```python
from build123d import *

# Parameters (mm, degrees)
BOSS_EXTRUDE1_DEPTH = 24
SKETCH2_R           = 5
BOSS_EXTRUDE2_DEPTH = 16
FILLET1_R           = 2
SKETCH4_W           = 5.41
SKETCH4_H           = 3.8
CUT_EXTRUDE1_DEPTH  = 20


with BuildPart() as part:
    # Sketch1 → Boss-Extrude1 (new body)
    with BuildSketch(Plane(origin=(0, 0, 0), x_dir=(0, 0, -1), z_dir=(1, 0, 0))):
        with BuildLine():
            Line((1.8, 31.882308546), (9.77686398, 36.487753113))
            Line((9.77686398, 36.487753113), (14.382308546, 28.510889132))
            ThreePointArc((14.382308546, 28.510889132), (15.7, 27.193197679), (17.5, 26.710889132))
            Line((17.5, 26.710889132), (26.710889132, 26.710889132))
            Line((26.710889132, 26.710889132), (26.710889132, 17.5))
            ThreePointArc((26.710889132, 17.5), (27.193197679, 15.7), (28.510889132, 14.382308546))
            Line((28.510889132, 14.382308546), (36.487753113, 9.77686398))
            Line((36.487753113, 9.77686398), (31.882308546, 1.8))
            ThreePointArc((31.882308546, 1.8), (31.4, 0), (31.882308546, -1.8))
            Line((31.882308546, -1.8), (36.487753113, -9.77686398))
            Line((36.487753113, -9.77686398), (28.510889132, -14.382308546))
            ThreePointArc((28.510889132, -14.382308546), (27.193197679, -15.7), (26.710889132, -17.5))
            Line((26.710889132, -17.5), (26.710889132, -26.710889132))
            Line((26.710889132, -26.710889132), (17.5, -26.710889132))
            ThreePointArc((17.5, -26.710889132), (15.7, -27.193197679), (14.382308546, -28.510889132))
            Line((14.382308546, -28.510889132), (9.77686398, -36.487753113))
            Line((9.77686398, -36.487753113), (1.8, -31.882308546))
            ThreePointArc((1.8, -31.882308546), (0, -31.4), (-1.8, -31.882308546))
            Line((-1.8, -31.882308546), (-9.77686398, -36.487753113))
            Line((-9.77686398, -36.487753113), (-14.382308546, -28.510889132))
            ThreePointArc((-14.382308546, -28.510889132), (-15.7, -27.193197679), (-17.5, -26.710889132))
            Line((-17.5, -26.710889132), (-26.710889132, -26.710889132))
            Line((-26.710889132, -26.710889132), (-26.710889132, -17.5))
            ThreePointArc((-26.710889132, -17.5), (-27.193197679, -15.7), (-28.510889132, -14.382308546))
            Line((-28.510889132, -14.382308546), (-36.487753113, -9.77686398))
            Line((-36.487753113, -9.77686398), (-31.882308546, -1.8))
            ThreePointArc((-31.882308546, -1.8), (-31.4, 0), (-31.882308546, 1.8))
            Line((-31.882308546, 1.8), (-36.487753113, 9.77686398))
            Line((-36.487753113, 9.77686398), (-28.510889132, 14.382308546))
            ThreePointArc((-28.510889132, 14.382308546), (-27.193197679, 15.7), (-26.710889132, 17.5))
            Line((-26.710889132, 17.5), (-26.710889132, 26.710889132))
            Line((-26.710889132, 26.710889132), (-17.5, 26.710889132))
            ThreePointArc((-17.5, 26.710889132), (-15.7, 27.193197679), (-14.382308546, 28.510889132))
            Line((-14.382308546, 28.510889132), (-9.77686398, 36.487753113))
            Line((-9.77686398, 36.487753113), (-1.8, 31.882308546))
            ThreePointArc((-1.8, 31.882308546), (0, 31.4), (1.8, 31.882308546))
        make_face()
    extrude(amount=BOSS_EXTRUDE1_DEPTH)

    # Sketch2 → Boss-Extrude2 (add)
    with BuildSketch(Plane(origin=(24, 0, 0), x_dir=(0, 0, -1), z_dir=(1, 0, 0))):
        Circle(SKETCH2_R)
    extrude(amount=BOSS_EXTRUDE2_DEPTH)

    # Fillet1
    fillet1_edges = [part.edges().sort_by_distance(p)[0] for p in [
        (24, 0, 5),
    ]]
    fillet(fillet1_edges, radius=FILLET1_R)

    # Sketch4 → Cut-Extrude1 (cut)
    with BuildSketch(Plane(origin=(40, 0, 0), x_dir=(0, 0, -1), z_dir=(1, 0, 0))):
        Rectangle(SKETCH4_W, SKETCH4_H)
    extrude(amount=-CUT_EXTRUDE1_DEPTH, mode=Mode.SUBTRACT)


solid = part.part
```
Can you work these out from the model? Positions are in its coordinate system, mm. A direction names the side the tool comes from. Round coordinates to 2 decimals unless told otherwise and drop trailing zeros. Order: outer loops, then holes, each group sorted by start corner. A loop starts at its lowest first (then second) coordinate and runs counter-clockwise, first axis right, second up.
(1) On a 3-axis mill with a long thin cutter (end or side, diameter ignored), from which of +Z, -Z, +X, -X, +Y, -Y can I reach the whole of each face in a straight line? I mean faces 4 (the face through (12, 22, -26.711)), 5 (the face through (12, -26.711, 22)), 6 (the face through (12, -26.711, -22)). Say none if no direction works.
Results are:
face 4: -Z, +X, -X, +Y
face 5: +Z, +X, -X, -Y
face 6: -Z, +X, -X, -Y
(2) If we section it at C-C (z = -23.5): Please give me the cut outline in (x, y), plus the area to 3 significant figures.
Results are:
outline: (0, -26.71) - (24, -26.71) - (24, 26.71) - (0, 26.71) - close
area: 1,280 mm2
(3) If we section it at A-A (y = 0): Please give me the cut outline in (x, z) (3 decimals).
Results are:
outline: (0, -31.4) - (24, -31.4) - (24, -7) arc R2 cw to (26, -5) - (40, -5) - (40, -2.705) - (20, -2.705) - (20, 2.705) - (40, 2.705) - (40, 5) - (26, 5) arc R2 cw to (24, 7) - (24, 31.4) - (0, 31.4) - close
(4) I'm going to push flat-ended pins straight in: pin 1 (2 mm diameter, centred on x = 4.5, z = -22, fed in from -Y); pin 2 (1.6 mm diameter, centred on x = 27.5, z = 0, fed in from -Y); pin 3 (3 mm diameter, centred on x = 27, y = 8.5, fed in from -Z); pin 4 (4.5 mm diameter, centred on x = 6, z = -20.5, fed in from +Y). Where does each tip first touch, or does it pass through?
Results are:
pin 1: stops at y = -26.71
pin 2: stops at y = -5
pin 3: passes through
pin 4: stops at y = 26.71
(5) We'd pull the mould along Y, two halves only. Please class faces 1 (the face through (30, -1.9, 0)), 2 (the face through (11.832, -27.206, 15.677)), 3 (the face through (11.832, 15.677, 27.206)): +Y half, -Y half, draft (parallel to the pull), parting line (faces both ways), or undercut.
Results are:
face 1: undercut
face 2: -Y half
face 3: +Y half
(6) If we section it at B-B (z = 0): Please give me the cut outline in (x, y), plus the area to 3 significant figures.
Results are:
outline: (0, -31.4) - (24, -31.4) - (24, -7) arc R2 cw to (26, -5) - (40, -5) - (40, -1.9) - (20, -1.9) - (20, 1.9) - (40, 1.9) - (40, 5) - (26, 5) arc R2 cw to (24, 7) - (24, 31.4) - (0, 31.4) - close
area: 1,590 mm2
(7) If I drill on L1, parallel to X at y = -20.5, z = 20.5; L2, parallel to Y at x = 13, z = -32; L3, parallel to Z at x = 13, y = 23.5, over which ranges is the centre line in solid material (lowest first)?
Results are:
L1: x = 0 to 24
L2: y = -12.37 to -2, 2 to 12.37
L3: z = -26.71 to 26.71
